from build123d import *

# Parameters (mm, degrees)
F0_W      = 40.25
F0_H      = 5.25
F1_DEPTH  = 77.5
F2_W      = 38.52346
F2_H      = 72.027471
F3_DEPTH  = 5
F4_W      = 41.75
F4_H      = 8.25
F5_DEPTH  = 1.5
F6_W      = 43.25
F6_H      = 8.25
F6_R      = 3.5
F6_W_2    = 13
F6_H_2    = 5
F7_DEPTH  = 2
F8_W      = 3.5
F8_H      = 18
F9_DEPTH  = 5
F11_DEPTH = 12.5


with BuildPart() as f1:
    # F0 (on Top) → F1 (new body)
    with BuildSketch(Plane.XY):
        with BuildLine():
            Line((-21.625, 3.375), (-21.625, -3.375))
            ThreePointArc((-21.625, -3.375), (-21.40533, -3.90533), (-20.875, -4.125))
            Line((-20.875, -4.125), (20.875, -4.125))
            ThreePointArc((20.875, -4.125), (21.40533, -3.90533), (21.625, -3.375))
            Line((21.625, -3.375), (21.625, 3.375))
            ThreePointArc((21.625, 3.375), (21.40533, 3.90533), (20.875, 4.125))
            Line((20.875, 4.125), (-20.875, 4.125))
            ThreePointArc((-20.875, 4.125), (-21.40533, 3.90533), (-21.625, 3.375))
        make_face()
        Rectangle(F0_W, F0_H, mode=Mode.SUBTRACT)
    extrude(amount=F1_DEPTH)

    # F2 (on face) → F3 (cut)
    with BuildSketch(Plane.XZ.offset(4.125)):
        with Locations((0.057188, 40.02151)):
            Rectangle(F2_W, F2_H)
    extrude(amount=-F3_DEPTH, mode=Mode.SUBTRACT)

    # F4 (on face) → F5 (join)
    with BuildSketch(Plane.XY.offset(77.5)):
        Rectangle(F4_W, F4_H)
        with BuildLine():
            add(Edge.make_bspline(
                [(18.290351, -0.923601), (18.290351, 1.241462), (13.790351, 0.158931), (9.290351, -0.923601), (13.790351, -2.006133), (18.290351, -3.088665), (18.290351, -0.923601)],
                knots=[0, 0, 0, 2.094395, 2.094395, 4.18879, 4.18879, 6.283185, 6.283185, 6.283185], degree=2, weights=[1, 0.5, 1, 0.5, 1, 0.5, 1]))
        make_face(mode=Mode.SUBTRACT)
    extrude(amount=F5_DEPTH)

    # F6 (on Top) → F7 (join)
    with BuildSketch(Plane.XY):
        Rectangle(F6_W, F6_H)
        with Locations((-17.708602, 0)):
            Circle(F6_R, mode=Mode.SUBTRACT)
        with Locations((13.390783, 0.038613)):
            Rectangle(F6_W_2, F6_H_2, mode=Mode.SUBTRACT)
    extrude(amount=-F7_DEPTH)

    # F8 (on face) → F9 (cut)
    with BuildSketch(Plane(origin=(-21.625, 0, 0), x_dir=(0, -1, 0), z_dir=(-1, 0, 0))):
        with Locations((0.002663, 65.263712)):
            Rectangle(F8_W, F8_H)
    extrude(amount=-F9_DEPTH, mode=Mode.SUBTRACT)

    # F10 (on Right) → F11 (join, symmetric)
    with BuildSketch(Plane.YZ):
        Polygon((7.875, 66.051362), (4.125, 66.051362), (4.125, 63.051362), (5.882013, 63.051362), (5.882013, 31.051362), (7.875, 31.051362), align=None)
    extrude(amount=F11_DEPTH, both=True)


solid = f1.part
Design review of the part built by this model. Coordinates are the model's own, in mm. A direction names the side the tool comes from. Give positions to 0.01 mm unless a question says otherwise; leave off trailing zeros. Order: outer loops, then holes, each group sorted by start corner. A loop starts at its lowest first (then second) coordinate and runs counter-clockwise, first axis right, second up. Notation, with made-up numbers: (55, 48.25) - (69, 48.25) arc R16 ccw to (69, 65.25) - close; hole circle Ø6 at (79, -17). An arc over 180 degrees is marked (long way). Use CSV: the item, a comma, the result in double quotes. Start each with the question number.
Q1. Machinability: for faces 1 (the face through (-19.5, -2.625, 21.3)), 2 (the face through (0, 5, 63.051)), 3 (the face through (-21, 0, 56.264)), 4 (the face through (-14.37, 1.05, -0.99)), 5 (the face through (0, -3, 4.008)), which of the approach directions +Z, -Z, +X, -X, +Y, -Y give a long, thin tool a straight path to every point of the face, cutting with its end or side? Answer none if there is none.
Q2. Draft analysis for pull direction Y (two halves, no side actions). For faces 6 (the face through (0, 7.875, 48)), 7 (the face through (-21.625, 0, 38)), 8 (the face through (0, 4.125, 39)), state which applies: pulls with the +Y half, pulls with the -Y half, needs draft (parallel to the pull), parting line crosses it, or undercut.
Q3. Take a section at B-B (x = -2). State the section outline as (y, z) points (3 decimals).
Q4. Take a section at A-A (z = 62). State the section outline as (x, y) points (3 decimals), and give its area (3 significant figures).
Q5. For P1, Ø1.6, axis at y = -1, z = 78, coming from the +X side (3 decimals); P2, Ø1, axis at x = -15, z = 50.5, coming from the -Y side (3 decimals); P3, Ø0.8, axis at y = -1, z = 78.5, coming from the -X side (3 decimals); P4, Ø1, axis at y = 5, z = 59.5, coming from the -X side, all flat-tipped, find the tip position at first contact; note any pin that passes through.
Q6. For line 1 (Z direction, x = -14.5, y = -2.75); line 2 (X direction, y = -1.75, z = 5) (3 decimals); line 3 (Z direction, x = -11, y = 1), list the stretches that pass through material, from the lowest coordinate up.
Q7. Take a section at C-C (z = 36.5). State the section outline as (x, y) points (3 decimals).
Calculated:
1,face 1,"none"
1,face 2,"-Z, +X, -X"
1,face 3,"-X"
1,face 4,"-Z"
1,face 5,"-Y"
2,face 6,"pulls with the +Y half"
2,face 7,"needs draft"
2,face 8,"undercut"
3,outline,"(-4.125, -2) - (4.125, -2) - (4.125, 63.051) - (5.882, 63.051) - (5.882, 31.051) - (7.875, 31.051) - (7.875, 66.051) - (4.125, 66.051) - (4.125, 79) - (-4.125, 79) - (-4.125, 76.035) - (-2.625, 76.035) - (-2.625, 77.5) - (2.625, 77.5) - (2.625, 0) - (-2.625, 0) - (-2.625, 4.008) - (-4.125, 4.008) - close"
4,outline,"(-21.625, -3.375) arc R0.75 ccw to (-20.875, -4.125) - (-19.205, -4.125) - (-19.205, -2.625) - (-20.125, -2.625) - (-20.125, -1.753) - (-21.625, -1.753) - close; (-21.625, 1.747) - (-20.125, 1.747) - (-20.125, 2.625) - (20.125, 2.625) - (20.125, -2.625) - (19.319, -2.625) - (19.319, -4.125) - (20.875, -4.125) arc R0.75 ccw to (21.625, -3.375) - (21.625, 3.375) arc R0.75 ccw to (20.875, 4.125) - (-20.875, 4.125) arc R0.75 ccw to (-21.625, 3.375) - close; (-12.5, 5.882) - (12.5, 5.882) - (12.5, 7.875) - (-12.5, 7.875) - close"
4,area,"132 mm²"
5,P1,"stops at x = 21.625"
5,P2,"stops at y = 2.625"
5,P3,"stops at x = -20.875"
5,P4,"passes through"
6,line 1,"z = -2 to 4.01, 76.04 to 79"
6,line 2,"x = -21.625 to -20.125, 20.125 to 21.625"
6,line 3,"z = -2 to 0, 77.5 to 79"
7,outline,"(-21.625, -3.375) arc R0.75 ccw to (-20.875, -4.125) - (-19.205, -4.125) - (-19.205, -2.625) - (-20.125, -2.625) - (-20.125, 2.625) - (20.125, 2.625) - (20.125, -2.625) - (19.319, -2.625) - (19.319, -4.125) - (20.875, -4.125) arc R0.75 ccw to (21.625, -3.375) - (21.625, 3.375) arc R0.75 ccw to (20.875, 4.125) - (-20.875, 4.125) arc R0.75 ccw to (-21.625, 3.375) - close; (-12.5, 5.882) - (12.5, 5.882) - (12.5, 7.875) - (-12.5, 7.875) - close"
